Autodesk Fusion 360 part; units mm, degrees
sketch "Sketch1" plane through (0, 0, 0) normal (0, 0, 1) x (1, 0, 0)
  line L0 (8.5, 2.25) -> (-8.5, 2.25)
  line L1 (-8.5, 2.25) -> (-8.5, -2.25)
  line L2 (-8.5, -2.25) -> (8.5, -2.25)
  line L3 (8.5, -2.25) -> (8.5, 2.25)
  line L4 (8.5, 2.25) -> (-8.5, -2.25) construction
  line L5 (-8.5, 2.25) -> (8.5, -2.25) construction
  dimension "d1" = 17
  dimension "d2" = 4.5
extrude "Extrude1" add sketch "Sketch1" along normal blind 12
sketch "Sketch2" plane through (0, 0, 12) normal (0, 0, 1) x (1, 0, 0)
  line L0 (8.5, -2.25) -> (8.5, 2.25)
  line L1 (8.5, 2.25) -> (-8.5, 2.25)
  line L2 (-8.5, 2.25) -> (-8.5, -2.25)
  line L3 (-8.5, -2.25) -> (8.5, -2.25)
  line L4 (3.9, 1.65) -> (-3.9, 1.65)
  line L5 (-3.9, 1.65) -> (-3.9, -1.15)
  line L6 (-3.9, -1.15) -> (3.9, -1.15)
  line L7 (3.9, -1.15) -> (3.9, 1.65)
  line L8 (3.9, 1.65) -> (-3.9, -1.15) construction
  line L9 (-3.9, 1.65) -> (3.9, -1.15) construction
  point P0 (0, 0.25)
  dimension "d5" = 7.8
  dimension "d6" = 2.8
  dimension "d7" = 0.6
extrude "Extrude2" add sketch "Sketch2" along normal blind 4 contours L4 L5 L6 L7
fillet "Fillet1" radius 1 4 edges at (-8.5, 2.25, 6) (-8.5, -2.25, 6) (8.5, -2.25, 6) (8.5, 2.25, 6)
fillet "Fillet2" radius 0.9 4 edges at (3.9, 1.65, 14) (-3.9, 1.65, 14) (3.9, -1.15, 14) (-3.9, -1.15, 14)
CAD build for the part. Positions are in the model's coordinates, mm. A direction names the side the tool comes from. Coordinates: 2 decimals unless noted, no trailing zeros. Loops run counter-clockwise (first coordinate to the right, second up) from the corner with the lowest first, then second, coordinate; pieces in that order, holes last. Notation, with made-up numbers: (-32.75, 36.5) - (18.25, 36.5) arc R21 ccw to (18.25, 47.5) - close; hole circle Ø10 at (76, -28.5). An arc over 180 degrees is marked (long way). Use one line per item in the form item = value. Start each with the question number.
1) Flat gauge pins, fed straight in: pin 1 (1.1 mm diameter, centred on y = 0, z = 13, fed in from +X); pin 2 (3 mm diameter, centred on x = -1, z = 14, fed in from -Y); pin 3 (4 mm diameter, centred on x = 2, z = 14.5, fed in from +Y). Where does each tip first touch, or does it go through?
2) Band-saw the part on B-B (y = 0.5). Give the cut face in (x, z), and give its area (3 significant figures).
3) Band-saw the part on A-A (z = 14). Give the cut face in (x, y), and give its area (3 significant figures).
4) Band-saw the part on C-C (x = 6.5). Give the cut face in (y, z), and give its area (3 significant figures).
5) Band-saw the part on D-D (y = -1.5). Give the cut face in (x, z), and give its area (3 significant figures).
6) Tool access for faces 1 (the face through (3.9, 0, 14)), 2 (the face through (0, 1.65, 14)), 3 (the face through (-3.9, 0, 14)), 4 (the face through (3.64, 1.38, 14.03)): list every direction of +Z, -Z, +X, -X, +Y, -Y with a clear straight run to the whole face (end or side of a thin tool).
7) Drill centre lines: L1, parallel to Y at x = 1, z = 12.25; L2, parallel to Z at x = -7, y = 2; L3, parallel to X at y = 0.2, z = 14.5. Where is each one in solid material? Low to high. Write a range as from..to.
Check values:
q1.pin_1 = 3.9
q1.pin_2 = -1.15
q1.pin_3 = 1.65
q2.outline = (-8.5, 0) - (8.5, 0) - (8.5, 12) - (3.9, 12) - (3.9, 16) - (-3.9, 16) - (-3.9, 12) - (-8.5, 12) - close
q2.area = 235 mm2
q3.outline = (-3.9, -0.25) arc R0.9 ccw to (-3, -1.15) - (3, -1.15) arc R0.9 ccw to (3.9, -0.25) - (3.9, 0.75) arc R0.9 ccw to (3, 1.65) - (-3, 1.65) arc R0.9 ccw to (-3.9, 0.75) - close
q3.area = 21.1 mm2
q4.outline = (-2.25, 0) - (2.25, 0) - (2.25, 12) - (-2.25, 12) - close
q4.area = 54.0 mm2
q5.outline = (-8.47, 0) - (8.47, 0) - (8.47, 12) - (-8.47, 12) - close
q5.area = 203 mm2
q6.face_1 = +Z, +X, +Y, -Y
q6.face_2 = +Z, +X, -X, +Y
q6.face_3 = +Z, -X, +Y, -Y
q6.face_4 = +Z, +X, +Y
q7.L1 = -1.15..1.65
q7.L2 = 0..12
q7.L3 = -3.9..3.9
